from build123d import *

# Parameters (mm, degrees)
SKETCH1_W           = 192.0875
SKETCH1_H           = 161.925
BOSS_EXTRUDE1_DEPTH = 3.175
SKETCH2_W           = 19.05
SKETCH2_H           = 3.175
BOSS_EXTRUDE2_DEPTH = 3.175
CUT_EXTRUDE1_DEPTH  = 128.724709611
FILLET1_R           = 0.508
CUT_EXTRUDE2_REACH  = 129.725
SKETCH4_R           = 1.6256
CUT_EXTRUDE3_REACH  = 129.725
SKETCH5_R           = 1.6


with BuildPart() as part:
    # Sketch1 → Boss-Extrude1 (new body)
    with BuildSketch(Plane(origin=(0, 0, 0), x_dir=(1, 0, 0), z_dir=(0, 1, 0))):
        Rectangle(SKETCH1_W, SKETCH1_H)
    extrude(amount=BOSS_EXTRUDE1_DEPTH)

    # Sketch2 → Boss-Extrude2 (add)
    with BuildSketch(Plane(origin=(0, 3.175, 0), x_dir=(1, 0, 0), z_dir=(0, 1, 0))):
        with Locations((-63.5, 82.55)):
            Rectangle(SKETCH2_W, SKETCH2_H)
        with Locations((63.5, 82.55)):
            Rectangle(SKETCH2_W, SKETCH2_H)
        with Locations((-63.5, -82.55)):
            Rectangle(SKETCH2_W, SKETCH2_H)
        with Locations((63.5, -82.55)):
            Rectangle(SKETCH2_W, SKETCH2_H)
    extrude(amount=-BOSS_EXTRUDE2_DEPTH)

    # Sketch3 → Cut-Extrude1 (cut, through all)
    with BuildSketch(Plane(origin=(0, 3.175, 0), x_dir=(1, 0, 0), z_dir=(0, 1, 0))):
        with BuildLine():
            Line((-57.15, 74.6125), (57.15, 74.6125))
            ThreePointArc((57.15, 74.6125), (63.5, 68.2625), (57.15, 61.9125))
            Line((57.15, 61.9125), (-57.15, 61.9125))
            ThreePointArc((-57.15, 61.9125), (-63.5, 68.2625), (-57.15, 74.6125))
        make_face()
    extrude(amount=-CUT_EXTRUDE1_DEPTH, mode=Mode.SUBTRACT)

    # Fillet1
    fillet1_edges = [part.edges().sort_by_distance(p)[0] for p in [
        (73.025, 1.5875, 80.9625),
        (53.975, 1.5875, 80.9625),
        (-53.975, 1.5875, 80.9625),
        (-73.025, 1.5875, 80.9625),
        (53.975, 1.5875, -80.9625),
        (73.025, 1.5875, -80.9625),
        (-53.975, 1.5875, -80.9625),
        (-73.025, 1.5875, -80.9625),
    ]]
    fillet(fillet1_edges, radius=FILLET1_R)

    # Sketch4 → Cut-Extrude2 (cut, up to next)
    with BuildSketch(Plane.XZ, mode=Mode.PRIVATE) as cut_extrude2_sk1:
        with Locations(Location((-82.7024, 51.9049, 0), (0, 0, 270))):
            Circle(SKETCH4_R)
    cut_extrude2_tool1 = extrude(cut_extrude2_sk1.sketch, amount=-CUT_EXTRUDE2_REACH, mode=Mode.PRIVATE) & part.part
    # Sketch4 → Cut-Extrude2 (cut, up to next)
    with BuildSketch(Plane.XZ, mode=Mode.PRIVATE) as cut_extrude2_sk2:
        with Locations(Location((-82.7024, 21.1201, 0), (0, 0, 270))):
            Circle(SKETCH4_R)
    cut_extrude2_tool2 = extrude(cut_extrude2_sk2.sketch, amount=-CUT_EXTRUDE2_REACH, mode=Mode.PRIVATE) & part.part
    # Sketch4 → Cut-Extrude2 (cut, up to next)
    with BuildSketch(Plane.XZ, mode=Mode.PRIVATE) as cut_extrude2_sk3:
        with Locations(Location((82.7024, 21.1201, 0), (0, 0, 270))):
            Circle(SKETCH4_R)
    cut_extrude2_tool3 = extrude(cut_extrude2_sk3.sketch, amount=-CUT_EXTRUDE2_REACH, mode=Mode.PRIVATE) & part.part
    # Sketch4 → Cut-Extrude2 (cut, up to next)
    with BuildSketch(Plane.XZ, mode=Mode.PRIVATE) as cut_extrude2_sk4:
        with Locations(Location((82.7024, 51.9049, 0), (0, 0, 270))):
            Circle(SKETCH4_R)
    cut_extrude2_tool4 = extrude(cut_extrude2_sk4.sketch, amount=-CUT_EXTRUDE2_REACH, mode=Mode.PRIVATE) & part.part
    add(cut_extrude2_tool1.solids().sort_by_distance((-82.7024, 0, 51.9049))[0], mode=Mode.SUBTRACT)
    add(cut_extrude2_tool2.solids().sort_by_distance((-82.7024, 0, 21.1201))[0], mode=Mode.SUBTRACT)
    add(cut_extrude2_tool3.solids().sort_by_distance((82.7024, 0, 21.1201))[0], mode=Mode.SUBTRACT)
    add(cut_extrude2_tool4.solids().sort_by_distance((82.7024, 0, 51.9049))[0], mode=Mode.SUBTRACT)

    # Sketch5 → Cut-Extrude3 (cut, up to next)
    with BuildSketch(Plane(origin=(0, 3.175, 0), x_dir=(1, 0, 0), z_dir=(0, 1, 0)), mode=Mode.PRIVATE) as cut_extrude3_sk1:
        with Locations(Location((66.1333, 1.8125, 0), (0, 0, 270))):
            Circle(SKETCH5_R)
    cut_extrude3_tool1 = extrude(cut_extrude3_sk1.sketch, amount=-CUT_EXTRUDE3_REACH, mode=Mode.PRIVATE) & part.part
    # Sketch5 → Cut-Extrude3 (cut, up to next)
    with BuildSketch(Plane(origin=(0, 3.175, 0), x_dir=(1, 0, 0), z_dir=(0, 1, 0)), mode=Mode.PRIVATE) as cut_extrude3_sk2:
        with Locations(Location((66.1333, 45.1125, 0), (0, 0, 270))):
            Circle(SKETCH5_R)
    cut_extrude3_tool2 = extrude(cut_extrude3_sk2.sketch, amount=-CUT_EXTRUDE3_REACH, mode=Mode.PRIVATE) & part.part
    # Sketch5 → Cut-Extrude3 (cut, up to next)
    with BuildSketch(Plane(origin=(0, 3.175, 0), x_dir=(1, 0, 0), z_dir=(0, 1, 0)), mode=Mode.PRIVATE) as cut_extrude3_sk3:
        with Locations(Location((-56.25, 45.1125, 0), (0, 0, 270))):
            Circle(SKETCH5_R)
    cut_extrude3_tool3 = extrude(cut_extrude3_sk3.sketch, amount=-CUT_EXTRUDE3_REACH, mode=Mode.PRIVATE) & part.part
    # Sketch5 → Cut-Extrude3 (cut, up to next)
    with BuildSketch(Plane(origin=(0, 3.175, 0), x_dir=(1, 0, 0), z_dir=(0, 1, 0)), mode=Mode.PRIVATE) as cut_extrude3_sk4:
        with Locations(Location((-56.25, 1.8125, 0), (0, 0, 270))):
            Circle(SKETCH5_R)
    cut_extrude3_tool4 = extrude(cut_extrude3_sk4.sketch, amount=-CUT_EXTRUDE3_REACH, mode=Mode.PRIVATE) & part.part
    add(cut_extrude3_tool1.solids().sort_by_distance((66.1333, 3.175, -1.8125))[0], mode=Mode.SUBTRACT)
    add(cut_extrude3_tool2.solids().sort_by_distance((66.1333, 3.175, -45.1125))[0], mode=Mode.SUBTRACT)
    add(cut_extrude3_tool3.solids().sort_by_distance((-56.25, 3.175, -45.1125))[0], mode=Mode.SUBTRACT)
    add(cut_extrude3_tool4.solids().sort_by_distance((-56.25, 3.175, -1.8125))[0], mode=Mode.SUBTRACT)


solid = part.part
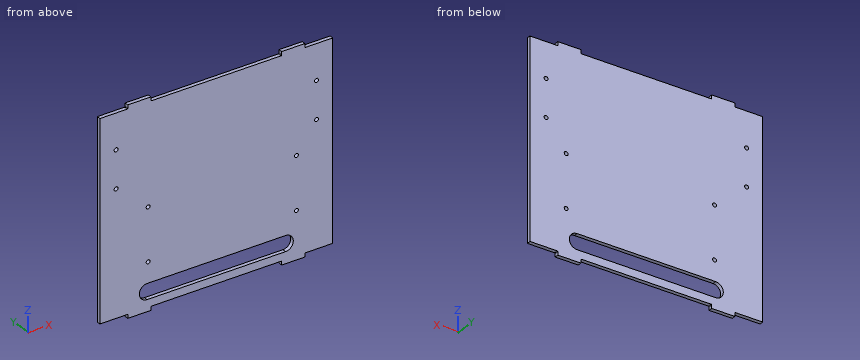
Build history of the part. All positions in model axes, mm. Round coordinates to 2 decimals unless told otherwise and drop trailing zeros. Use CSV: the item, a comma, the result in double quotes. Start each with the question number.
(1) Drill centre lines: probe 1 along Z at (x, y) = (39, 2.6); probe 2 along Z at (x, y) = (74.5, 1.05); probe 3 along X at (y, z) = (1.75, 51). Where is each one in solid material? Low to high.
(2) Cut at A-A on y = 2.5. State how many separate pieces and enclosed holes the cut face has, then the cut area to 3 significant figures.
(3) Flat gauge pins, fed straight in: P1, Ø1.9, axis at x = -56.25, z = -45.11, coming from the +Y side; P2, Ø0.8, axis at y = 1, z = 83.5, coming from the +X side (3 decimals); P3, Ø1, axis at x = 26, y = 1.5, coming from the -Z side. Where does each tip first touch, or does it go through?
Findings:
1,probe 1,"z = -80.96 to -74.61, -61.91 to 80.96"
1,probe 2,"z = -80.96 to 80.96"
1,probe 3,"x = -96.04 to -84.05, -81.35 to 81.35, 84.05 to 96.04"
2,separate pieces,"1"
2,enclosed holes,"9"
2,area,"29,700 mm^2"
3,P1,"passes through"
3,P2,"stops at x = 73.025"
3,P3,"stops at z = -80.96"
